Input: part model. Units: mm. Frame: model coordinates. A direction names the side the tool comes from. Give positions to 0.01 mm unless a question says otherwise; leave off trailing zeros. Write each loop counter-clockwise with the first axis right and the second up, starting at its lowest first coordinate (ties: lowest second). Pieces come first, ordered by that corner, then holes. Notation, with made-up numbers: M 61.25,41.5 L 97.25,41.5 A22 cw 97.25,73.5 Z; hole C -7,80.5 d7. An arc over 180 degrees is marked long. Use CSV: the item, a comma, the result in double quotes. Start each with the question number.
from build123d import *

# Parameters (mm, degrees)
BOX003_W        = 10
BOX003_H        = 2
BOX003_DEPTH    = 3
BOX002_W        = 10
BOX002_H        = 2
BOX002_DEPTH    = 3
BOX004_W        = 2
BOX004_H        = 11
BOX004_DEPTH    = 3
CHAMFER002_SIZE = 1
CHAMFER003_SIZE = 0.5


with BuildPart() as cube003:
    # Box003 → Box003 (new body)
    with BuildSketch(Plane(origin=(15.5, 13, 0), x_dir=(1, 0, 0), z_dir=(0, 0, 1))):
        with Locations((5, 1)):
            Rectangle(BOX003_W, BOX003_H)
    extrude(amount=BOX003_DEPTH)


with BuildPart() as cube002:
    # Box002 → Box002 (new body)
    with BuildSketch(Plane(origin=(15.5, 0, 0), x_dir=(1, 0, 0), z_dir=(0, 0, 1))):
        with Locations((5, 1)):
            Rectangle(BOX002_W, BOX002_H)
    extrude(amount=BOX002_DEPTH)


with BuildPart() as chamfer003:
    # Box004 → Box004 (new body)
    with BuildSketch(Plane(origin=(15.5, 2, 0), x_dir=(1, 0, 0), z_dir=(0, 0, 1))):
        with Locations((1, 5.5)):
            Rectangle(BOX004_W, BOX004_H)
    extrude(amount=BOX004_DEPTH)

    # Fusion002: union Cube003, Cube002
    add(cube003.part)
    add(cube002.part)

    # Chamfer002
    chamfer002_edges = [chamfer003.edges().sort_by_distance(p)[0] for p in [
        (15.5, 0, 1.5),
        (15.5, 15, 1.5),
        (17.5, 2, 1.5),
        (17.5, 13, 1.5),
    ]]
    chamfer(chamfer002_edges, length=CHAMFER002_SIZE)

    # Chamfer003
    chamfer003_edges = [chamfer003.edges().sort_by_distance(p)[0] for p in [
        (15.5, 1, 1.5),
        (16.5, 0, 1.5),
        (15.5, 14, 1.5),
        (16.5, 15, 1.5),
    ]]
    chamfer(chamfer003_edges, length=CHAMFER003_SIZE)


solid = chamfer003.part
Q1. Section A-A, the plane x = 24.75. Return the cut outline in (y, z), and give its area (3 significant figures).
Q2. Material intervals for L1, parallel to Y at x = 21.25, z = 0.3; L2, parallel to X at y = 4.5, z = 2.65; L3, parallel to Y at x = 18.25, z = 0.6, sorted ascending. Write a range as [from, to].
Q3. Pull-direction query (Y, two-part tool) for faces 1 (the flat face through (18, 2.5, 1.5)), 2 (the flat face through (22, 13, 1)), 3 (the flat face through (16.579, 0.174, 1.479)), 4 (the flat face through (15.68, 13.93, 1.48)); classes: released by +Y, released by -Y, zero draft, split by the parting line, or undercut.
Q4. Set-up query: faces 5 (the flat face through (17, 8, 0)), 6 (the flat face through (18, 12.5, 1.5)). Return all of +Z, -Z, +X, -X, +Y, -Y with unobstructed straight access to the full face (end or side cutting, diameter ignored); none if empty.
Q5. Section C-C, the plane x = 18.25. Return the cut outline in (y, z).
Q6. First-contact query: pin 1 Ø1.5 at (y, z) = (9.5, 2) entering from +X. Flat tip, straight axial feed; report the tip coordinate or a pass-through.
Q7. Section B-B, the plane z = 2.65. Return the cut outline in (x, y).
Q8. Section D-D, the plane y = 11. Return the cut outline in (x, z), and give its area (3 significant figures).
Check result:
1,outline,"M 0,0 L 2,0 L 2,3 L 0,3 Z; M 13,0 L 15,0 L 15,3 L 13,3 Z"
1,area,"12.0 mm²"
2,L1,"y = [0, 2], [13, 15]"
2,L2,"x = [15.5, 17.5]"
2,L3,"y = [0, 2.25], [12.75, 15]"
3,face 1,"undercut"
3,face 2,"undercut"
3,face 3,"released by -Y"
3,face 4,"released by +Y"
4,face 5,"-Z, +X, -X, +Y, -Y"
4,face 6,"+Z, -Z, +X"
5,outline,"M 0,0 L 2.25,0 L 2.25,3 L 0,3 Z; M 12.75,0 L 15,0 L 15,3 L 12.75,3 Z"
6,pin 1,"stops at x = 17.5"
7,outline,"M 15.5,1.5 L 15.85,0.65 L 16.15,0.35 L 17,0 L 25.5,0 L 25.5,2 L 18.5,2 L 17.5,3 L 17.5,12 L 18.5,13 L 25.5,13 L 25.5,15 L 17,15 L 16.15,14.65 L 15.85,14.35 L 15.5,13.5 Z"
8,outline,"M 15.5,0 L 17.5,0 L 17.5,3 L 15.5,3 Z"
8,area,"6.00 mm²"
